Could you check a few things on this model? Use its own coordinates, in mm. Coordinates: 2 decimals unless noted, no trailing zeros. Write each loop counter-clockwise with the first axis right and the second up, starting at its lowest first coordinate (ties: lowest second). Pieces come first, ordered by that corner, then holes. Notation, with made-up numbers: (38, 55.5) - (43, 55.5) arc R35 ccw to (43, 90.5) - close; hole circle Ø10 at (-2.5, -8.75). An arc over 180 degrees is marked (long way). Answer as a JSON object with one key per item and string values. Group by question number.
1) If we section it at C-C (x = 8): Write out the boundary of the cut face in (y, z), plus the area to 3 significant figures.
2) Will these pins go through, and if not, where does the flat tip stop? pin 1 Ø10 at (x, y) = (30, 43) entering from -Z; pin 2 Ø2 at (y, z) = (15.5, 3.5) entering from +X; pin 3 Ø1.9 at (x, z) = (9.5, 4.5) entering from -Y; pin 4 Ø3 at (y, z) = (20, 0.5) entering from +X.
3) If we section it at D-D (y = 20): Write out the boundary of the cut face in (x, z), plus the area to 3 significant figures.
4) If we section it at A-A (y = 51.5): Write out the boundary of the cut face in (x, z).
5) If we section it at B-B (z = 2.5): Write out the boundary of the cut face in (x, y) (3 decimals).
6) Please list where these lines run through material, in increasing order: line 1 along X through (y, z) = (50, 4.5); line 2 along Y through (x, z) = (18.5, 6.25); line 3 along X through (y, z) = (-10.5, 4.5).
```python
from build123d import *

# Parameters (mm, degrees)
F1_DEPTH = 6.35
F2_R     = 25.4
F3_R     = 12.7
F4_R     = 25.4
F5_R     = 4.7752
F7_D     = 12.7
F9_D     = 6.35
F11_D    = 6.35


with BuildPart() as f1:
    # F0 (on Top) → F1 (new body)
    with BuildSketch(Plane.XY):
        Polygon((55.1337133169, 65.8959785044), (-52.8162866831, 65.8959785044), (-52.8162866831, -23.0040214956), (-27.4162866831, -23.0040214956), (-27.4162866831, 27.7959785044), (55.1337133169, 27.7959785044), align=None)
    extrude(amount=F1_DEPTH)

    # F2
    f2_edges = [f1.edges().sort_by_distance(p)[0] for p in [
        (-52.816287, 65.895979, 3.175),
    ]]
    fillet(f2_edges, radius=F2_R)

    # F3
    f3_edges = [f1.edges().sort_by_distance(p)[0] for p in [
        (55.133713, 65.895979, 3.175),
        (55.133713, 27.795979, 3.175),
    ]]
    fillet(f3_edges, radius=F3_R)

    # F4
    f4_edges = [f1.edges().sort_by_distance(p)[0] for p in [
        (-27.416287, 27.795979, 3.175),
    ]]
    fillet(f4_edges, radius=F4_R)

    # F5
    f5_edges = [f1.edges().sort_by_distance(p)[0] for p in [
        (-27.416287, -23.004021, 3.175),
        (-52.816287, -23.004021, 3.175),
    ]]
    fillet(f5_edges, radius=F5_R)

    # F7 (through all)
    with Locations(Plane(origin=(0, 0, 0), x_dir=(1, 0, 0), z_dir=(0, 0, -1))):
        with Locations((39.2587133169, -46.8459785044)):
            Hole(F7_D / 2)

    # F9 (through all)
    with Locations(Plane(origin=(0, 0, 0), x_dir=(1, 0, 0), z_dir=(0, 0, -1))):
        with Locations((-40.1162866831, 10.3040214956)):
            Hole(F9_D / 2)

    # F11 (through all)
    with Locations(Plane(origin=(0, 0, 0), x_dir=(1, 0, 0), z_dir=(0, 0, -1))):
        with Locations((-40.1162866831, -50.0209785044)):
            Hole(F11_D / 2)


solid = f1.part
```
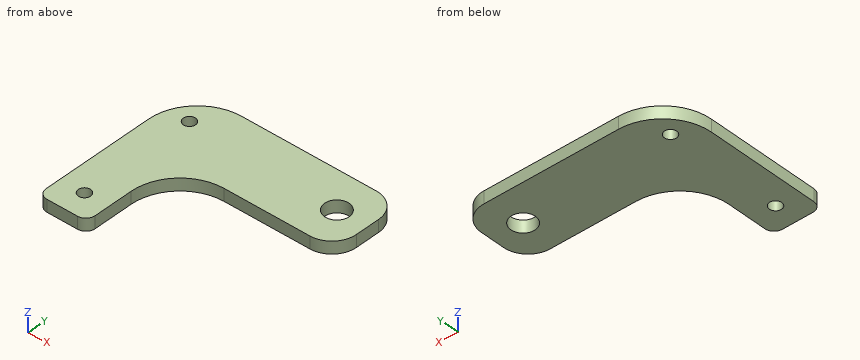
Here are the results:
{
 "1": {"outline": "(27.8, 0) - (65.9, 0) - (65.9, 6.35) - (27.8, 6.35) - close", "area": "242 mm²"},
 "2": {"pin 1": "stops at z = 0", "pin 2": "stops at x = -23.14", "pin 3": "stops at y = 27.8", "pin 4": "stops at x = -18.76"},
 "3": {"outline": "(-52.82, 0) - (-20.33, 0) - (-20.33, 6.35) - (-52.82, 6.35) - close", "area": "206 mm²"},
 "4": {"outline": "(-50.31, 0) - (-42.93, 0) - (-42.93, 6.35) - (-50.31, 6.35) - close; (-37.31, 0) - (34.94, 0) - (34.94, 6.35) - (-37.31, 6.35) - close; (43.58, 0) - (55.13, 0) - (55.13, 6.35) - (43.58, 6.35) - close"},
 "5": {"outline": "(-52.816, -18.229) arc R4.775 ccw to (-48.041, -23.004) - (-32.191, -23.004) arc R4.775 ccw to (-27.416, -18.229) - (-27.416, 2.396) arc R25.4 cw to (-2.016, 27.796) - (42.434, 27.796) arc R12.7 ccw to (55.134, 40.496) - (55.134, 53.196) arc R12.7 ccw to (42.434, 65.896) - (-27.416, 65.896) arc R25.4 ccw to (-52.816, 40.496) - close; hole circle Ø6.35 at (-40.116, -10.304); hole circle Ø6.35 at (-40.116, 50.021); hole circle Ø12.7 at (39.259, 46.846)"},
 "6": {"line 1": "x = -50.97 to -43.29, -36.94 to 33.75, 44.77 to 55.13", "line 2": "y = 27.8 to 65.9", "line 3": "x = -52.82 to -43.29, -36.95 to -27.42"}
}
